Could you check a few things on this model? Use its own coordinates, in mm. Face numbers are marked on the shaded views. A direction names the side the tool comes from. Give positions to 0.01 mm unless a question says otherwise; leave off trailing zeros. Order: outer loops, then holes, each group sorted by start corner. A loop starts at its lowest first (then second) coordinate and runs counter-clockwise, first axis right, second up.
(1) Will these pins go through, and if not, where does the flat tip stop? pin 1 (2 mm diameter, centred on x = 29, y = 107, fed in from -Z) (3 decimals); pin 2 (6 mm diameter, centred on x = -17, y = 51, fed in from +Z) (3 decimals); pin 3 (14.5 mm diameter, centred on x = 61.96, z = -61.96, fed in from +Y); pin 4 (7.5 mm diameter, centred on x = -61.96, z = -61.96, fed in from +Y).
(2) Imagine slicing it at C-C, the plane y = 50.5. Write out the boundary of the cut face in (x, z) (3 decimals), then the cut area to 3 significant figures.
(3) Imagine slicing it at A-A, the plane x = 0. State how many separate pieces and enclosed holes the cut face has, then the cut area to 3 significant figures.
(4) If we mould it in two halves opening along X, with no side actions, what happens to the marked faces 6, 7 and 8? For each: released by +X, released by -X, zero draft, split by the parting line, or undercut.
(5) If I drill on probe 1 along Z at (x, y) = (-38, 7); probe 2 along Y at (x, z) = (0, 21) (3 decimals); probe 3 along X at (y, z) = (76, -31) (3 decimals), over which ranges is the centre line in solid material (lowest first)?
(6) Imagine slicing it at D-D, the plane z = 23.5. Write out the boundary of the cut face in (x, y) (3 decimals).
(7) Imagine slicing it at B-B, the plane z = 0. Write out the boundary of the cut face in (x, y).
(8) On a 3-axis mill with a long thin cutter (end or side, diameter ignored), from which of +Z, -Z, +X, -X, +Y, -Y can I reach the whole of each face in a straight line? I mean the marked faces 1, 2, 3, 4 and 5. Say none if no direction works.
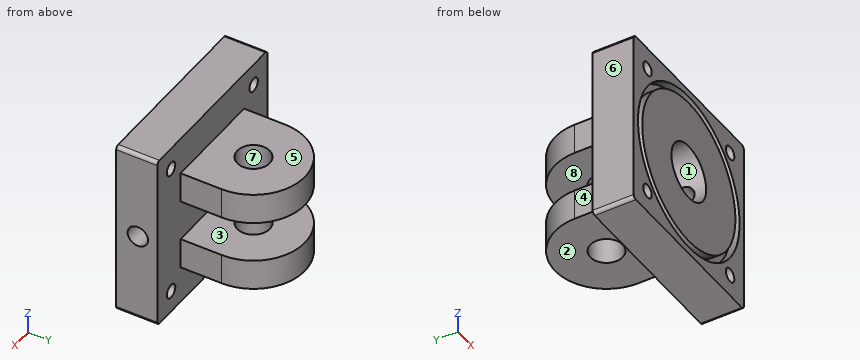
from build123d import *

# Parameters (mm, degrees)
SKETCH1_R                         = 6.35
BOSS_EXTRUDE1_DEPTH               = 38.1
BOSS_EXTRUDE2_START               = -34.925
SKETCH2_R                         = 15
BOSS_EXTRUDE2_DEPTH               = 28.575
SKETCH3_R                         = 26
CUT_EXTRUDE1_DEPTH                = 36.83
SKETCH4_R                         = 76.2
SKETCH4_R_2                       = 69.85
CUT_EXTRUDE2_DEPTH                = 8
F_1_2_14_NPSM_TAPPED_HOLE1_REACH  = 224.273
F_1_2_14_NPSM_TAPPED_HOLE1_BORE_R = 9.4869


with BuildPart() as part:
    # Sketch1 → Boss-Extrude1 (new body)
    with BuildSketch(Plane(origin=(0, 0, 0), x_dir=(1, 0, 0), z_dir=(0, 1, 0))):
        with BuildLine():
            Line((-79.375, -82.55), (79.375, -82.55))
            ThreePointArc((79.375, -82.55), (81.62006403, -81.62006403), (82.55, -79.375))
            Line((82.55, -79.375), (82.55, 79.375))
            ThreePointArc((82.55, 79.375), (81.62006403, 81.62006403), (79.375, 82.55))
            Line((79.375, 82.55), (-79.375, 82.55))
            ThreePointArc((-79.375, 82.55), (-81.62006403, 81.62006403), (-82.55, 79.375))
            Line((-82.55, 79.375), (-82.55, -79.375))
            ThreePointArc((-82.55, -79.375), (-81.62006403, -81.62006403), (-79.375, -82.55))
        make_face()
        with Locations(Location((61.963767235, 61.963767235, 0), (0, 0, 90))):
            Circle(SKETCH1_R, mode=Mode.SUBTRACT)
        with Locations(Location((61.963767235, -61.963767235, 0), (0, 0, 90))):
            Circle(SKETCH1_R, mode=Mode.SUBTRACT)
        with Locations(Location((-61.963767235, -61.963767235, 0), (0, 0, 90))):
            Circle(SKETCH1_R, mode=Mode.SUBTRACT)
        with Locations(Location((-61.963767235, 61.963767235, 0), (0, 0, 90))):
            Circle(SKETCH1_R, mode=Mode.SUBTRACT)
    extrude(amount=BOSS_EXTRUDE1_DEPTH)

    # Sketch2 → Boss-Extrude2 (add)
    with BuildSketch(Plane.XY.offset(82.55).offset(BOSS_EXTRUDE2_START)):
        with BuildLine():
            Line((-47.625, 38.1), (-47.625, 76.2))
            ThreePointArc((-47.625, 76.2), (0, 123.825), (47.625, 76.2))
            Line((47.625, 76.2), (47.625, 38.1))
            Line((47.625, 38.1), (-47.625, 38.1))
        make_face()
        with Locations((0, 76.2)):
            Circle(SKETCH2_R, mode=Mode.SUBTRACT)
    boss_extrude2 = extrude(amount=-BOSS_EXTRUDE2_DEPTH)

    # Mirror1: Boss-Extrude2 across plane
    add(boss_extrude2.mirror(Plane.XY))

    # Sketch3 → Cut-Extrude1 (cut)
    with BuildSketch(Plane.XZ):
        with Locations(Location((0, 0, 0), (0, 0, 270))):
            Circle(SKETCH3_R)
    extrude(amount=-CUT_EXTRUDE1_DEPTH, mode=Mode.SUBTRACT)

    # Sketch4 → Cut-Extrude2 (cut)
    with BuildSketch(Plane.XZ):
        with Locations(Location((0, 0, 0), (0, 0, 270))):
            Circle(SKETCH4_R)
        with Locations(Location((0, 0, 0), (0, 0, 270))):
            Circle(SKETCH4_R_2, mode=Mode.SUBTRACT)
    extrude(amount=-CUT_EXTRUDE2_DEPTH, mode=Mode.SUBTRACT)

    # 1/2-14 NPSM Tapped Hole1 bore → 1/2-14 NPSM Tapped Hole1 (cut, up to next)
    with BuildSketch(Plane(origin=(82.55, 0, 0), x_dir=(0, 0, -1), z_dir=(1, 0, 0)), mode=Mode.PRIVATE) as f_1_2_14_npsm_tapped_hole1_sk1:
        with Locations((0, 20.05)):
            Circle(F_1_2_14_NPSM_TAPPED_HOLE1_BORE_R)
    f_1_2_14_npsm_tapped_hole1_tool1 = extrude(f_1_2_14_npsm_tapped_hole1_sk1.sketch, amount=-F_1_2_14_NPSM_TAPPED_HOLE1_REACH, mode=Mode.PRIVATE) & part.part
    add(f_1_2_14_npsm_tapped_hole1_tool1.solids().sort_by_distance((82.55, 20.05, 0))[0], mode=Mode.SUBTRACT)


solid = part.part
Answer block:
1. pin 1: stops at z = -47.625
1. pin 2: stops at z = 47.625
1. pin 3: stops at y = 38.1
1. pin 4: passes through
2. outline: (-47.625, -47.625) - (47.625, -47.625) - (47.625, -19.05) - (-47.625, -19.05) - close; (-47.625, 19.05) - (47.625, 19.05) - (47.625, 47.625) - (-47.625, 47.625) - close
2. area: 5,440 mm2
3. separate pieces: 3
3. enclosed holes: 0
3. area: 7,460 mm2
4. face 6: released by -X
4. face 7: undercut
4. face 8: zero draft
5. probe 1: z = -82.55 to -66.05, -58.61 to 58.61, 66.05 to 82.55
5. probe 2: y = 36.83 to 61.2, 91.2 to 123.825
5. probe 3: x = -47.625 to -14.999, 14.999 to 47.625
6. outline: (-82.55, 0) - (-72.486, 0) - (-72.486, 8) - (-65.778, 8) - (-65.778, 0) - (-11.124, 0) - (-11.124, 36.83) - (11.124, 36.83) - (11.124, 0) - (65.778, 0) - (65.778, 8) - (72.486, 8) - (72.486, 0) - (82.55, 0) - (82.55, 38.1) - (47.625, 38.1) - (47.625, 76.2) arc R47.625 ccw to (-47.625, 76.2) - (-47.625, 38.1) - (-82.55, 38.1) - close; hole circle Ø30 at (0, 76.2)
7. outline: (-82.55, 0) - (-76.2, 0) - (-76.2, 8) - (-69.85, 8) - (-69.85, 0) - (-26, 0) - (-26, 36.83) - (26, 36.83) - (26, 29.54) - (82.55, 29.54) - (82.55, 38.1) - (-82.55, 38.1) - close; (26, 0) - (69.85, 0) - (69.85, 8) - (76.2, 8) - (76.2, 0) - (82.55, 0) - (82.55, 10.56) - (26, 10.56) - close
8. face 1: -Y
8. face 2: -Z, +X, -X, +Y
8. face 3: +X, -X, +Y
8. face 4: +Z, -Z, -X, +Y
8. face 5: +Z, +X, -X, +Y
